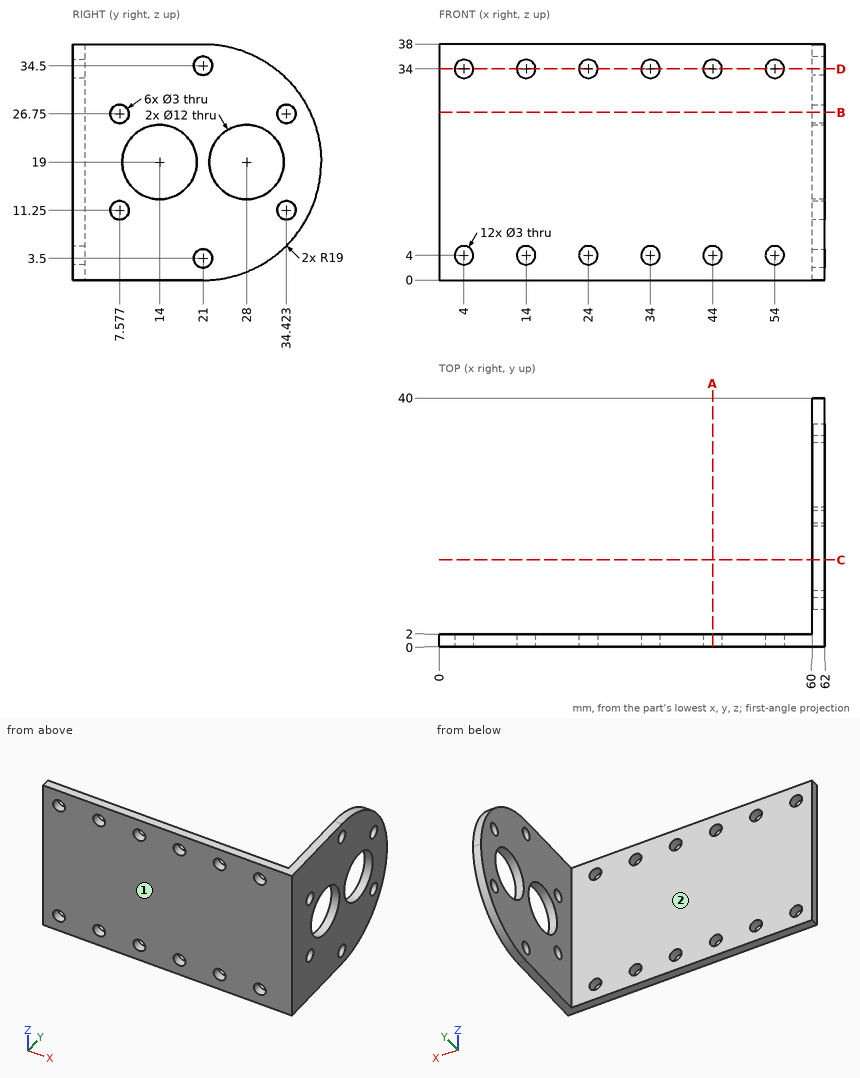
Study the drawing (mm; zero at the part's minimum x, y, z) and answer. A direction names the side the tool comes from. Give positions to 0.01 mm unless a question says otherwise; leave off trailing zeros. Order: outer loops, then holes, each group sorted by start corner. A loop starts at its lowest first (then second) coordinate and runs counter-clockwise, first axis right, second up. Notation, with made-up numbers: M 45,-17.5 L 84,-17.5 A10 cw 84,-11.5 Z; hole C 82,8.5 d4. An arc over 180 degrees is marked long. Put each result on its own line as item: value. Start each with the question number.
Item 1: Find the intervals of material crossed by line 1 along Z through (x, y) = (54, 0.7); line 2 along X through (y, z) = (7.5, 23.5); line 3 along Y through (x, z) = (17, 27.5), in increasing order.
Item 2: The part is cut by section B-B, the plane z = 27. Determine the outline of the cut face in (x, y) (1 decimal).
Item 3: The part is cut by section A-A, the plane x = 44. Determine the outline of the cut face in (y, z).
Item 4: The part is cut by section D-D, the plane z = 34. State how many separate pieces and enclosed holes the cut face has.
Item 5: Which of the six approach directions +Z, -Z, +X, -X, +Y, -Y give full straight-line access (tool end or side, diameter ignored) to the marked faces 1 and 2?
Item 6: The part is cut by section C-C, the plane y = 14. Determine the outline of the cut face in (x, z).
Item 7: Flat-ended cylindrical pins translate along their axes: P1, Ø1, axis at y = 32.5, z = 23.5, coming from the -X side; P2, Ø1.5, axis at x = 21, z = 29.5, coming from the +Y side. Find the tip coordinate at first contact, or state that the pin passes through.
Answer key:
1. line 1: z = 0 to 2.5, 5.5 to 32.5, 35.5 to 38
1. line 2: x = 60 to 62
1. line 3: y = 0 to 2
2. outline: M 0,0 L 62,0 L 62,6.1 L 60,6.1 L 60,2 L 0,2 Z; M 60,9.1 L 62,9.1 L 62,32.9 L 60,32.9 Z; M 60,35.9 L 62,35.9 L 62,38.2 L 60,38.2 Z
3. outline: M 0,0 L 2,0 L 2,2.5 L 0,2.5 Z; M 0,5.5 L 2,5.5 L 2,32.5 L 0,32.5 Z; M 0,35.5 L 2,35.5 L 2,38 L 0,38 Z
4. separate pieces: 8
4. enclosed holes: 0
5. face 1: +Z, -Z, +X, -X, -Y
5. face 2: +Z, -Z, -X, +Y
6. outline: M 60,0 L 62,0 L 62,13 L 60,13 Z; M 60,25 L 62,25 L 62,38 L 60,38 Z
7. P1: stops at x = 60
7. P2: stops at y = 2
